Could you check a few things on this model? Use its own coordinates, in mm. A direction names the side the tool comes from. Give positions to 0.01 mm unless a question says otherwise; leave off trailing zeros. Write each loop counter-clockwise with the first axis right and the second up, starting at its lowest first coordinate (ties: lowest second). Pieces come first, ordered by that corner, then holes. Notation, with made-up numbers: M -15.5,71 L 27.5,71 A17 ccw 27.5,94 Z; hole C 52.5,-10 d7. An arc over 180 degrees is marked long. Use one line per item in the form item = value.
from build123d import *

# Parameters (mm, degrees)
BOSS_EXTRUDE1_DEPTH = 10
BOSS_EXTRUDE2_DEPTH = 10
SKETCH4_R           = 1.6
CUT_EXTRUDE1_DEPTH  = 10
SKETCH5_R           = 3
SKETCH5_R_2         = 1.6
CUT_EXTRUDE2_DEPTH  = 10


with BuildPart() as part:
    # Sketch2 → Boss-Extrude1 (new body)
    with BuildSketch(Plane(origin=(0, 0, 0), x_dir=(0, 0, -1), z_dir=(1, 0, 0))):
        with BuildLine():
            Line((-8, 0), (-1.6, 0))
            ThreePointArc((-1.6, 0), (0, 1.6), (1.6, 0))
            Line((1.6, 0), (8, 0))
            ThreePointArc((8, 0), (0, 8), (-8, 0))
        make_face()
    extrude(amount=BOSS_EXTRUDE1_DEPTH)

    # Sketch3 → Boss-Extrude2 (add)
    with BuildSketch(Plane.ZY):
        with BuildLine():
            Line((-8, 0), (-2.6, 0))
            ThreePointArc((-2.6, 0), (0, 2.6), (2.6, 0))
            Line((2.6, 0), (8, 0))
            ThreePointArc((8, 0), (0, 8), (-8, 0))
        make_face()
    extrude(amount=BOSS_EXTRUDE2_DEPTH)

    # Sketch4 → Cut-Extrude1 (cut)
    with BuildSketch(Plane.XZ):
        with Locations((-5, 5.3)):
            Circle(SKETCH4_R)
        with Locations((5, 5.3)):
            Circle(SKETCH4_R)
        with Locations((-5, -5.3)):
            Circle(SKETCH4_R)
        with Locations((5, -5.3)):
            Circle(SKETCH4_R)
    extrude(amount=-CUT_EXTRUDE1_DEPTH, mode=Mode.SUBTRACT)

    # Sketch5 → Cut-Extrude2 (cut)
    with BuildSketch(Plane(origin=(0, 4, 0), x_dir=(-1, 0, 0), z_dir=(0, -1, 0))):
        with Locations((-5, 5.3)):
            Circle(SKETCH5_R)
        with Locations((-5, 5.3)):
            Circle(SKETCH5_R_2, mode=Mode.SUBTRACT)
        with Locations((5, 5.3)):
            Circle(SKETCH5_R)
        with Locations((5, 5.3)):
            Circle(SKETCH5_R_2, mode=Mode.SUBTRACT)
        with Locations((5, -5.3)):
            Circle(SKETCH5_R)
        with Locations((-5, -5.3)):
            Circle(SKETCH5_R)
    extrude(amount=-CUT_EXTRUDE2_DEPTH, mode=Mode.SUBTRACT)


solid = part.part
1) For faces 1 (the flat face through (5.04, 4, 3.55)), 2 (the cylindrical face through (4.792, 1.972, -3.714)), 3 (the flat face through (0, 2, 0)), which set-ups out of +Z, -Z, +X, -X, +Y, -Y let a thin tool reach every point of the face, with its end or its side?
Checked values:
face_1 = +Y
face_2 = +Y, -Y
face_3 = -X, -Y
2) I want a section at C-C, the plane y = 3.75. Please give me the cut outline in (x, z), plus the area to 3 significant figures.
Checked values:
outline = M -10,-7.07 L 10,-7.07 L 10,7.07 L -10,7.07 Z; hole C -5,-5.3 d3.2; hole C -5,5.3 d3.2; hole C 5,-5.3 d3.2; hole C 5,5.3 d3.2
area = 250 mm2
3) For pin 1 Ø8 at (x, z) = (5, 5.3) entering from +Y; pin 2 Ø1.4 at (x, z) = (-6, 5.5) entering from +Y; pin 3 Ø3 at (x, z) = (0.5, -4.5) entering from +Y; pin 4 Ø2.5 at (x, z) = (-5, -5.3) entering from +Y, each with a flat end and sliding along its axis, tell me the tip position at first contact or that it passes through.
Checked values:
pin_1 = 7.89
pin_2 = 4
pin_3 = 7.42
pin_4 = through
4) Thinking about a two-plate mould opening in Z: for faces 4 (the cylindrical face through (0, 8, 0)), 5 (the cylindrical face through (5.1, 5.4, -2.3)), 6 (the flat face through (-10, 4, 0)), which applies, released by +Z, released by -Z, zero draft, split by the parting line, or undercut?
Checked values:
face_4 = split by the parting line
face_5 = undercut
face_6 = zero draft
5) I want a section at D-D, the plane z = -4. Please give me the cut outline in (x, y), plus the area to 3 significant figures.
Checked values:
outline = M -10,0 L -5.93,0 L -5.93,4 L -7.7,4 L -7.7,6.93 L -10,6.93 Z; M -4.07,0 L 4.07,0 L 4.07,4 L 2.3,4 L 2.3,6.93 L -2.3,6.93 L -2.3,4 L -4.07,4 Z; M 5.93,0 L 10,0 L 10,6.93 L 7.7,6.93 L 7.7,4 L 5.93,4 Z
area = 92.0 mm2
6) I want a section at A-A, the plane x = 5. Count the separate pieces of the cut face and the enclosed holes in it, plus the area to 3 significant figures.
Checked values:
separate_pieces = 3
enclosed_holes = 0
area = 49.5 mm2
7) If I drill on L1, parallel to X at y = 2.4, z = -5.3; L2, parallel to X at y = 4.9, z = -5.3; L3, parallel to Z at x = 5, y = 2.25, over which ranges is the centre line in solid material (lowest first)?
Checked values:
L1 = -10 to -6.6, -3.4 to 3.4, 6.6 to 10
L2 = -10 to -8, -2 to 2, 8 to 10
L3 = -7.68 to -6.9, -3.7 to 3.7, 6.9 to 7.68
8) I want a section at B-B, the plane z = 0. Please give me the cut outline in (x, y), plus the area to 3 significant figures.
Checked values:
outline = M -10,2.6 L 0,2.6 L 0,1.6 L 10,1.6 L 10,8 L -10,8 Z
area = 118 mm2
